Autodesk Inventor part; units mm, degrees
ref_plane "YZ Plane" through (0, 0, 0) normal (1, 0, 0) x (0, 1, 0)
ref_plane "XZ Plane" through (0, 0, 0) normal (0, 1, 0) x (-1, 0, 0)
ref_plane "XY Plane" through (0, 0, 0) normal (0, 0, 1) x (1, 0, 0)
sketch "스케치1" plane through (0, 0, 0) normal (0, 0, 1) x (1, 0, 0)
  line L0 (0, 0) -> (0, 800)
  line L1 (0, 800) -> (100, 800)
  line L2 (100, 800) -> (100, 960)
  line L3 (100, 960) -> (400, 960)
  line L4 (400, 960) -> (400, 800)
  line L5 (400, 800) -> (500, 800)
  line L6 (500, 800) -> (500, 0)
  line L7 (500, 0) -> (0, 0)
  line L8 (390, 950) -> (110, 950)
  line L9 (110, 950) -> (110, 790)
  line L10 (110, 790) -> (10, 790)
  line L11 (10, 790) -> (10, 10)
  line L12 (10, 10) -> (490, 10)
  line L13 (490, 10) -> (490, 790)
  line L14 (490, 790) -> (390, 790)
  line L15 (390, 790) -> (390, 950)
  line L16 (10, 280) -> (200, 280)
  line L17 (200, 280) -> (200, 290)
  line L18 (200, 290) -> (10, 290)
  line L19 (10, 290) -> (10, 280)
  line L20 (490, 280) -> (300, 280)
  line L21 (300, 280) -> (300, 290)
  line L22 (300, 290) -> (490, 290)
  line L23 (490, 290) -> (490, 280)
  dimension "d0" = 800
  dimension "d1" = 100
  dimension "d2" = 160
  dimension "d3" = 300
  dimension "d4" = 160
  dimension "d5" = 100
  dimension "d6" = 800
  dimension "d7" = 10
  dimension "d8" = 190
  dimension "d9" = 10
  dimension "d10" = 190
  dimension "d11" = 10
  dimension "d12" = 500
extrude "돌출1" add sketch "스케치1" along normal blind 500 contours L0 L1 L2 L3 L4 L5 L6 L7 | L13 L20 L21 L22 | L18 L17 L16 L11
sketch "스케치2" plane through (0, 0, 0) normal (0, 0, -1) x (-1, 0, 0)
  line L0 (-390, 790) -> (-390, 950)
  line L1 (-390, 950) -> (-110, 950)
  line L2 (-110, 950) -> (-110, 790)
  line L3 (-110, 790) -> (-10, 790)
  line L4 (-10, 790) -> (-10, 290)
  line L5 (-200, 290) -> (-10, 290)
  line L6 (-200, 280) -> (-200, 290)
  line L7 (-10, 280) -> (-200, 280)
  line L8 (-10, 280) -> (-10, 10)
  line L9 (-10, 10) -> (-490, 10)
  line L10 (-490, 10) -> (-490, 280)
  line L11 (-300, 280) -> (-490, 280)
  line L12 (-300, 290) -> (-300, 280)
  line L13 (-490, 290) -> (-300, 290)
  line L14 (-490, 290) -> (-490, 790)
  line L15 (-490, 790) -> (-390, 790)
  line L16 (0, 0) -> (0, 800)
  line L17 (0, 800) -> (-100, 800)
  line L18 (-100, 800) -> (-100, 960)
  line L19 (-100, 960) -> (-400, 960)
  line L20 (-400, 960) -> (-400, 800)
  line L21 (-400, 800) -> (-500, 800)
  line L22 (-500, 800) -> (-500, 0)
  line L23 (-500, 0) -> (0, 0)
extrude "돌출2" add sketch "스케치2" along normal blind 10 contours L0 L1 L2 L3 L4 L5 L6 L7 L8 L9 L10 L11 L12 L13 L14 L15 | L23 L22 L21 L20 L19 L18 L17 L16
sketch "스케치4" plane through (110, 950, 500) normal (0, -1, 0) x (1, 0, 0)
  line L0 (-10, 0) -> (-10, -510)
  line L1 (290, 0) -> (290, -510)
  line L2 (-10, -510) -> (290, -510)
  point P0 (-110, -500)
  point P1 (140, -390)
  point P2 (140, -450)
  dimension "d18" = 150
  dimension "d28" = 60
  dimension "d29" = 120
hole "구멍1" at (250, 950, 110) at (250, 950, 50) direction (0, 1, 0) diameter 10 end through all
properties part number "Space"
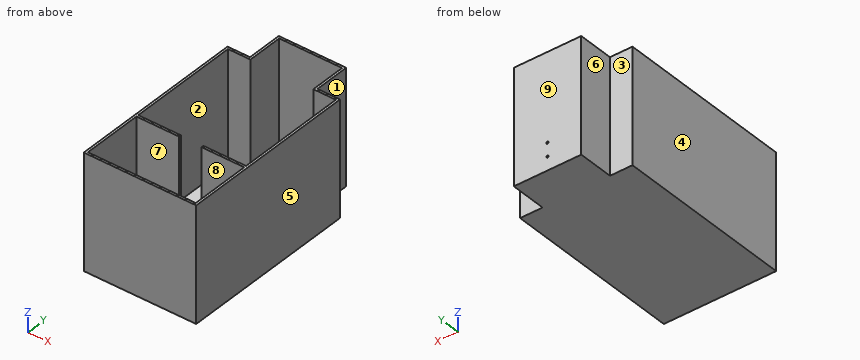
Model file for the job. Use its own axes, mm. Face numbers are marked on the shaded views. A direction names the side the tool comes from. Give positions to 0.01 mm unless a question says otherwise; leave off trailing zeros. Order: outer loops, then holes, each group sorted by start corner. A loop starts at its lowest first (then second) coordinate and runs counter-clockwise, first axis right, second up. Notation, with made-up numbers: (71.5, 0.25) -> (116.5, 0.25) arc R24 ccw to (116.5, 12.25) -> close; hole circle Ø10 at (38.25, 1.25). An arc over 180 degrees is marked (long way). Use CSV: the item, a comma, the result in double quotes.
1. Drop a flat-ended pin along its axis: pin 1 (6 mm diameter, centred on x = 273.5, y = 434, fed in from +Z). Give the stop position or say it passes through.
Outcome:
pin 1,"z = 0"
2. Band-saw the part on D-D, the plane y = 818.5. Give the cut face in (x, z), then the cut area to 3 significant figures.
Outcome:
outline,"(100, -10) -> (400, -10) -> (400, 500) -> (390, 500) -> (390, 0) -> (110, 0) -> (110, 500) -> (100, 500) -> close"
area,"13,000 mm²"
3. Band-saw the part on C-C, the plane y = 214.5. Give the cut face in (x, z).
Outcome:
outline,"(0, -10) -> (500, -10) -> (500, 500) -> (490, 500) -> (490, 0) -> (10, 0) -> (10, 500) -> (0, 500) -> close"
4. 3-axis set-ups, long thin cutter, end or side, ignore diameter. For the marked faces 1, 2, 3, 4 and 5: which of +Z, -Z, +X, -X, +Y, -Y reach the whole face in a straight line?
Outcome:
face 1,"+Z, -Z, +X, +Y"
face 2,"+Z"
face 3,"+Z, -Z, -X, +Y"
face 4,"+Z, -Z, -X, +Y, -Y"
face 5,"+Z, -Z, +X, +Y, -Y"
5. Mould opens along Y. For the marked faces 6, 7, 8 and 9 say: +Y half, -Y half, draft (parallel to the pull), parting line (faces both ways), or undercut.
Outcome:
face 6,"draft"
face 7,"undercut"
face 8,"undercut"
face 9,"+Y half"
6. Drill centre lines: line 1 along Y through (x, z) = (442.5, 406.5); line 2 along Y through (x, z) = (398.5, 212); line 3 along Z through (x, y) = (250, 956). Where is each one in solid material? Low to high. Write a range as from..to.
Outcome:
line 1,"0..10, 280..290, 790..800"
line 2,"0..10, 280..290, 790..960"
line 3,"-10..45, 55..105, 115..500"
7. Band-saw the part on B-B, the plane x = 39.5. Give the cut face in (y, z), then the cut area to 3 significant figures.
Outcome:
outline,"(0, -10) -> (800, -10) -> (800, 500) -> (790, 500) -> (790, 0) -> (290, 0) -> (290, 500) -> (280, 500) -> (280, 0) -> (10, 0) -> (10, 500) -> (0, 500) -> close"
area,"23,000 mm²"
8. Band-saw the part on A-A, the plane z = 202.5. Give the cut face in (x, y), then the cut area to 3 significant figures.
Outcome:
outline,"(0, 0) -> (500, 0) -> (500, 800) -> (400, 800) -> (400, 960) -> (100, 960) -> (100, 800) -> (0, 800) -> close; hole (10, 10) -> (490, 10) -> (490, 280) -> (300, 280) -> (300, 290) -> (490, 290) -> (490, 790) -> (390, 790) -> (390, 950) -> (110, 950) -> (110, 790) -> (10, 790) -> (10, 290) -> (200, 290) -> (200, 280) -> (10, 280) -> close"
area,"32,600 mm²"
